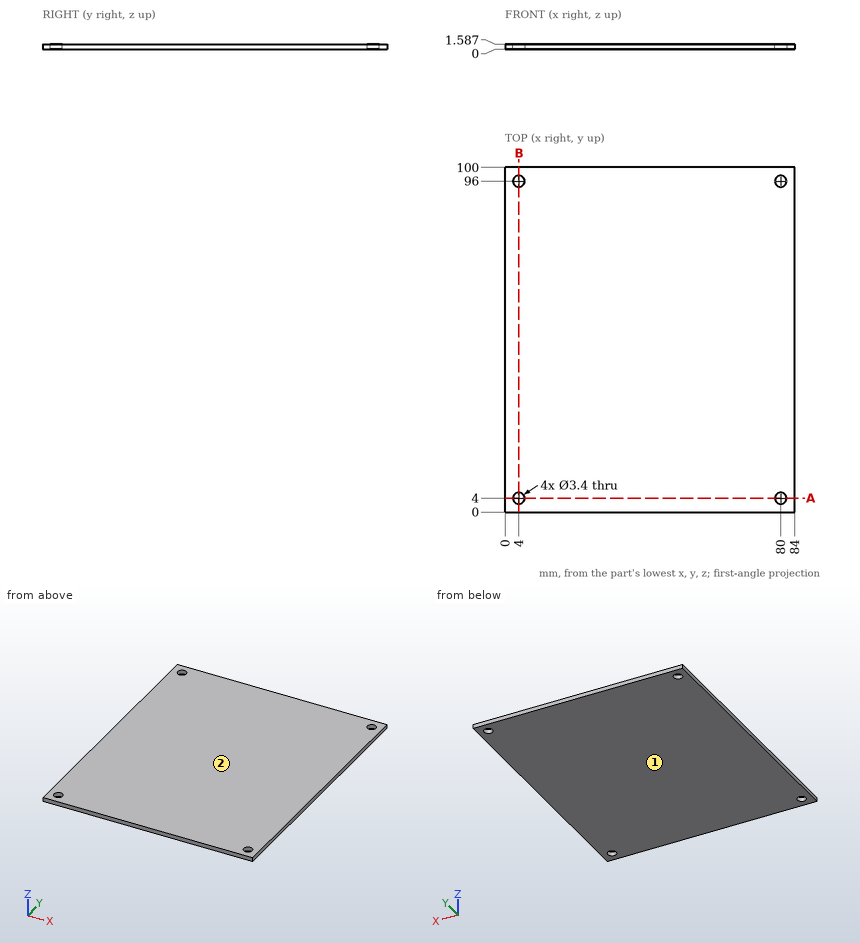
Check sheet for the drawn part. Datum: minimum x, y, z corner. Units: mm. Coordinates: 2 decimals unless noted, no trailing zeros. Loops run counter-clockwise (first coordinate to the right, second up) from the corner with the lowest first, then second, coordinate; pieces in that order, holes last. Notation, with made-up numbers: (-14, -0.75) - (13, -0.75) arc R10 ccw to (13, 15.25) - close; hole circle Ø11 at (-30, 25). An arc over 180 degrees is marked (long way). Put each result on its own line as item: value.
Item 1: Draft check along Z on the marked faces 1 and 2. Enter one of: pulls with the +Z half, pulls with the -Z half, needs draft (parallel to the pull), parting line crosses it, or undercut.
Conclusion:
face 1: pulls with the -Z half
face 2: pulls with the +Z half
Item 2: Section check B-B (x = 4). Enter the section's corners in (y, z).
Conclusion:
outline: (0, 0) - (2.3, 0) - (2.3, 1.59) - (0, 1.59) - close; (5.7, 0) - (94.3, 0) - (94.3, 1.59) - (5.7, 1.59) - close; (97.7, 0) - (100, 0) - (100, 1.59) - (97.7, 1.59) - close
Item 3: Section check A-A (y = 4). Enter the section's corners in (x, z).
Conclusion:
outline: (0, 0) - (2.3, 0) - (2.3, 1.59) - (0, 1.59) - close; (5.7, 0) - (78.3, 0) - (78.3, 1.59) - (5.7, 1.59) - close; (81.7, 0) - (84, 0) - (84, 1.59) - (81.7, 1.59) - close
Item 4: Scan lines: line 1 along Y through (x, z) = (80, 0.85); line 2 along X through (y, z) = (96, 0.75). Record each from-to range of solid material in increasing order.
Conclusion:
line 1: y = 0 to 2.3, 5.7 to 94.3, 97.7 to 100
line 2: x = 0 to 2.3, 5.7 to 78.3, 81.7 to 84
